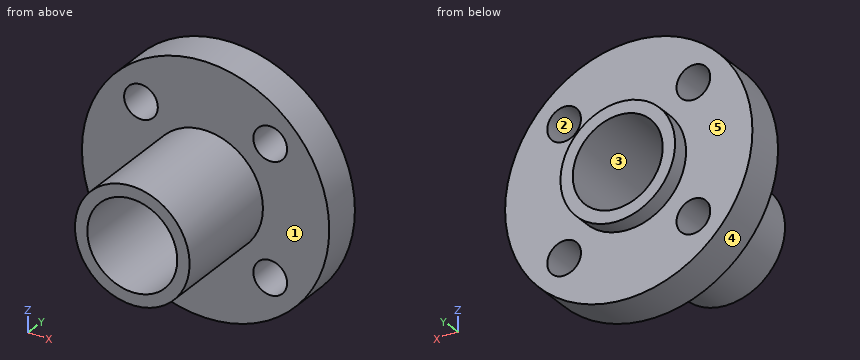
```python
from build123d import *

# Parameters (mm, degrees)
SKETCH1_R           = 11
SKETCH1_R_2         = 4
BOSS_EXTRUDE1_DEPTH = 3.5
SKETCH2_R           = 5.1
SKETCH2_R_2         = 4
BOSS_EXTRUDE2_DEPTH = 1.5
SKETCH3_R           = 5.1
SKETCH3_R_2         = 4
BOSS_EXTRUDE3_DEPTH = 10
CUT_EXTRUDE1_REACH  = 15.5
SKETCH4_R           = 1.5


with BuildPart() as part:
    # Sketch1 → Boss-Extrude1 (new body)
    with BuildSketch(Plane(origin=(0, 0, 0), x_dir=(1, 0, 0), z_dir=(0, 1, 0))):
        Circle(SKETCH1_R)
        Circle(SKETCH1_R_2, mode=Mode.SUBTRACT)
    extrude(amount=BOSS_EXTRUDE1_DEPTH)

    # Sketch2 → Boss-Extrude2 (add)
    with BuildSketch(Plane(origin=(0, 3.5, 0), x_dir=(1, 0, 0), z_dir=(0, 1, 0))):
        Circle(SKETCH2_R)
        Circle(SKETCH2_R_2, mode=Mode.SUBTRACT)
    extrude(amount=BOSS_EXTRUDE2_DEPTH)

    # Sketch3 → Boss-Extrude3 (add)
    with BuildSketch(Plane.XZ):
        Circle(SKETCH3_R)
        Circle(SKETCH3_R_2, mode=Mode.SUBTRACT)
    extrude(amount=BOSS_EXTRUDE3_DEPTH)

    # Sketch4 → Cut-Extrude1 (cut, up to next)
    with BuildSketch(Plane(origin=(0, 3.5, 0), x_dir=(1, 0, 0), z_dir=(0, 1, 0)), mode=Mode.PRIVATE) as cut_extrude1_sk1:
        with Locations((-5.75, 5.75)):
            Circle(SKETCH4_R)
    cut_extrude1_tool1 = extrude(cut_extrude1_sk1.sketch, amount=-CUT_EXTRUDE1_REACH, mode=Mode.PRIVATE) & part.part
    add(cut_extrude1_tool1.solids().sort_by_distance((-5.75, 3.5, -5.75))[0], mode=Mode.SUBTRACT)
    # Sketch4 → Cut-Extrude1 (cut, up to next)
    with BuildSketch(Plane(origin=(0, 3.5, 0), x_dir=(1, 0, 0), z_dir=(0, 1, 0)), mode=Mode.PRIVATE) as cut_extrude1_sk2:
        with Locations((5.75, 5.75)):
            Circle(SKETCH4_R)
    cut_extrude1_tool2 = extrude(cut_extrude1_sk2.sketch, amount=-CUT_EXTRUDE1_REACH, mode=Mode.PRIVATE) & part.part
    add(cut_extrude1_tool2.solids().sort_by_distance((5.75, 3.5, -5.75))[0], mode=Mode.SUBTRACT)
    # Sketch4 → Cut-Extrude1 (cut, up to next)
    with BuildSketch(Plane(origin=(0, 3.5, 0), x_dir=(1, 0, 0), z_dir=(0, 1, 0)), mode=Mode.PRIVATE) as cut_extrude1_sk3:
        with Locations((5.75, -5.75)):
            Circle(SKETCH4_R)
    cut_extrude1_tool3 = extrude(cut_extrude1_sk3.sketch, amount=-CUT_EXTRUDE1_REACH, mode=Mode.PRIVATE) & part.part
    add(cut_extrude1_tool3.solids().sort_by_distance((5.75, 3.5, 5.75))[0], mode=Mode.SUBTRACT)
    # Sketch4 → Cut-Extrude1 (cut, up to next)
    with BuildSketch(Plane(origin=(0, 3.5, 0), x_dir=(1, 0, 0), z_dir=(0, 1, 0)), mode=Mode.PRIVATE) as cut_extrude1_sk4:
        with Locations((-5.75, -5.75)):
            Circle(SKETCH4_R)
    cut_extrude1_tool4 = extrude(cut_extrude1_sk4.sketch, amount=-CUT_EXTRUDE1_REACH, mode=Mode.PRIVATE) & part.part
    add(cut_extrude1_tool4.solids().sort_by_distance((-5.75, 3.5, 5.75))[0], mode=Mode.SUBTRACT)


solid = part.part
```
Geometry: final body of the model. Coordinates: model frame, mm. Face numbers are marked on the shaded views. A direction names the side the tool comes from. Give positions to 0.01 mm unless a question says otherwise; leave off trailing zeros. Loops run counter-clockwise (first coordinate to the right, second up) from the corner with the lowest first, then second, coordinate; pieces in that order, holes last. Notation, with made-up numbers: (84.25, -26.75) -> (118.25, -26.75) arc R16 ccw to (118.25, -11.75) -> close; hole circle Ø3 at (61.25, -9.5). An arc over 180 degrees is marked (long way). Use one line per item in the form item = value.
Item 1: Section query C-C on y = 0.5. Output: boundary loops of the cut face in (x, z), and give its area (3 significant figures).
A:
outline = circle Ø22 at (0, 0); hole circle Ø3 at (-5.75, -5.75); hole circle Ø3 at (-5.75, 5.75); hole circle Ø8 at (0, 0); hole circle Ø3 at (5.75, -5.75); hole circle Ø3 at (5.75, 5.75)
area = 302 mm^2
Item 2: Access query for the marked faces 1 and 2. Directions: +Z, -Z, +X, -X, +Y, -Y. A direction counts if a zero-diameter tool reaches every point of the face in a straight line with its end or side. Return the directions, or none.
A:
face_1 = -Y
face_2 = +Y, -Y
Item 3: Line query: probe 1 along X at (y, z) = (1, -6); probe 2 along X at (y, z) = (2, -5.75). Output: solid intervals per line, ascending.
A:
probe_1 = -9.22 to -7.23, -4.27 to 4.27, 7.23 to 9.22
probe_2 = -9.38 to -7.25, -4.25 to 4.25, 7.25 to 9.38
Item 4: Section query D-D on z = -5.75. Output: boundary loops of the cut face in (x, y), and give its area (3 significant figures).
A:
outline = (-9.38, 0) -> (-7.25, 0) -> (-7.25, 3.5) -> (-9.38, 3.5) -> close; (-4.25, 0) -> (4.25, 0) -> (4.25, 3.5) -> (-4.25, 3.5) -> close; (7.25, 0) -> (9.38, 0) -> (9.38, 3.5) -> (7.25, 3.5) -> close
area = 44.6 mm^2
Item 5: Pin query (flat end, axial travel): P1, Ø4, axis at x = 5.75, z = -5.75, coming from the +Y side; P2, Ø4, axis at x = 8, y = 1, coming from the -Z side; P3, Ø2, axis at x = -0.5, y = -7.5, coming from the +Z side; P4, Ø1.8, axis at x = 5.75, z = 5.75, coming from the -Y side. Return the tip coordinate at first contact, or that it passes through.
A:
P1 = 3.5
P2 = -9.22
P3 = 5.1
P4 = through
Item 6: Section query A-A on x = 0. Output: boundary loops of the cut face in (y, z).
A:
outline = (-10, -5.1) -> (0, -5.1) -> (0, -11) -> (3.5, -11) -> (3.5, -5.1) -> (5, -5.1) -> (5, -4) -> (-10, -4) -> close; (-10, 4) -> (5, 4) -> (5, 5.1) -> (3.5, 5.1) -> (3.5, 11) -> (0, 11) -> (0, 5.1) -> (-10, 5.1) -> close
Item 7: Section query B-B on z = 0. Output: boundary loops of the cut face in (x, y).
A:
outline = (-11, 0) -> (-5.1, 0) -> (-5.1, -10) -> (-4, -10) -> (-4, 5) -> (-5.1, 5) -> (-5.1, 3.5) -> (-11, 3.5) -> close; (4, -10) -> (5.1, -10) -> (5.1, 0) -> (11, 0) -> (11, 3.5) -> (5.1, 3.5) -> (5.1, 5) -> (4, 5) -> close
Item 8: Draft query along Z for the marked faces 3, 4 and 5. Return one class per face: pulls with the +Z half, pulls with the -Z half, needs draft (parallel to the pull), parting line crosses it, or undercut.
A:
face_3 = undercut
face_4 = parting line crosses it
face_5 = needs draft
